Verification items for this drawing (mm, ordinates from the low corner). A direction names the side the tool comes from. Round coordinates to 2 decimals unless told otherwise and drop trailing zeros. Order: outer loops, then holes, each group sorted by start corner. A loop starts at its lowest first (then second) coordinate and runs counter-clockwise, first axis right, second up. Notation, with made-up numbers: M 17,66.25 L 42,66.25 A6 cw 42,76.25 Z; hole C -1,6 d4. An arc over 180 degrees is marked long. One line per item, written item: value. Start each with the question number.
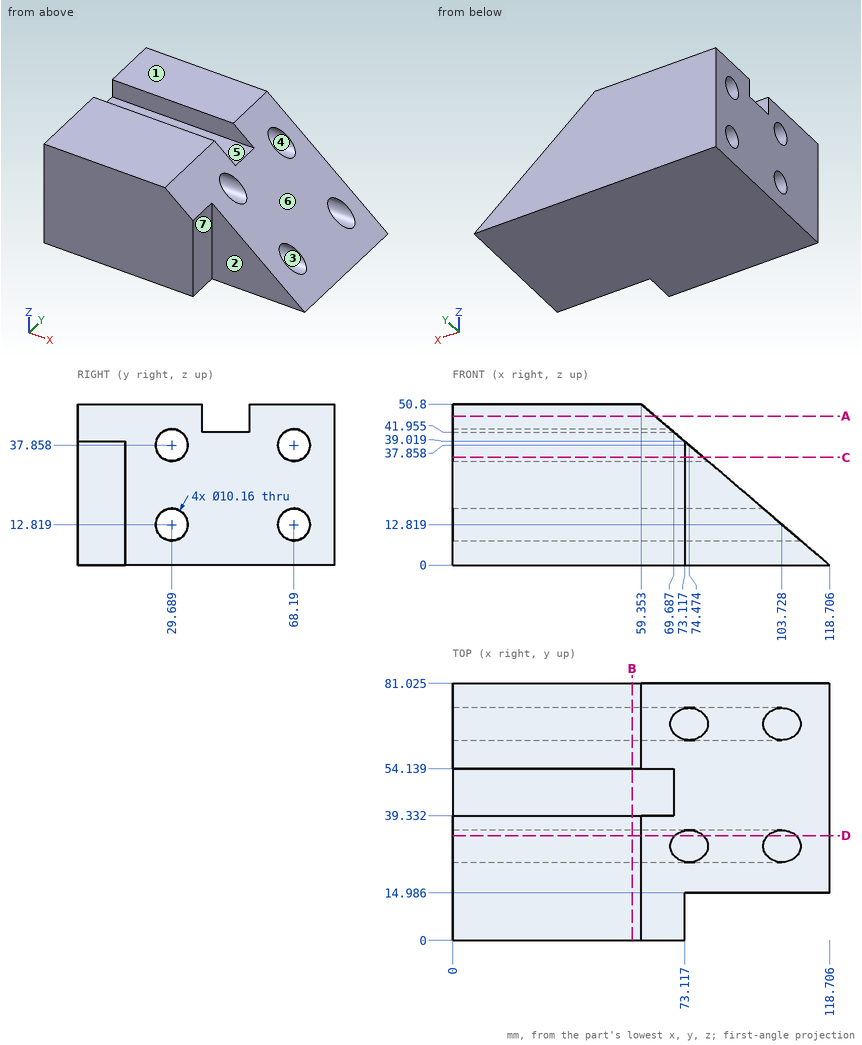
1. Section check A-A (z = 47). Record the cut outline in (x, y) (1 decimal).
2. Draft check along Z on the marked faces 1, 2, 3 and 4. Enter one of: released by +Z, released by -Z, zero draft, split by the parting line, or undercut.
3. Tool access check on the marked faces 5, 6 and 7. Record the directions out of +Z, -Z, +X, -X, +Y, -Y that give a thin tool (end or side, any length) a straight path to the whole face; none if there is none.
4. Depth check by flat-ended pin: pin 1 (19.5 mm diameter, centred on x = 90.5, z = 22.5, fed in from -Y); pin 2 (10 mm diameter, centred on x = 29, y = 29, fed in from -Z); pin 3 (2 mm diameter, centred on x = 60.5, y = 54, fed in from +Z) (1 decimal); pin 4 (1.5 mm diameter, centred on x = 84, y = 40.5, fed in from +Z) (1 decimal). Enter the tip coordinate at first touch or a pass-through.
5. Section check C-C (z = 34). Record the cut outline in (x, y) (1 decimal), and give its area (3 significant figures).
6. Scan lines: line 1 along Z through (x, y) = (37, 29) (1 decimal); line 2 along Z through (x, y) = (38.5, 70.5) (1 decimal); line 3 along X through (y, z) = (5.5, 39) (1 decimal). Record each from-to range of solid material in increasing order.
7. Section check D-D (y = 33). Record the cut outline in (x, z) (1 decimal), and give its area (3 significant figures).
8. Section check B-B (x = 56.5). Record the cut outline in (y, z) (1 decimal), and give its area (3 significant figures).
Geometry check:
1. outline: M 0,0 L 63.8,0 L 63.8,39.3 L 0,39.3 Z; M 0,54.1 L 63.8,54.1 L 63.8,81 L 0,81 Z
2. face 1: released by +Z
2. face 2: zero draft
2. face 3: undercut
2. face 4: undercut
3. face 5: +Z, +X, -X
3. face 6: +Z, +X, +Y, -Y
3. face 7: +Z, -Z, +X, -Y
4. pin 1: stops at y = 14.99
4. pin 2: stops at z = 0
4. pin 3: stops at z = 50.7
4. pin 4: stops at z = 30.3
5. outline: M 0,0 L 73.1,0 L 73.1,15 L 79,15 L 79,26.4 L 0,26.4 Z; M 0,33 L 79,33 L 79,64.9 L 0,64.9 Z; M 0,71.5 L 79,71.5 L 79,81 L 0,81 Z
5. area: 5,270 mm²
6. line 1: z = 0 to 7.8, 17.9 to 32.8, 42.9 to 50.8
6. line 2: z = 0 to 8.3, 17.3 to 33.3, 42.4 to 50.8
6. line 3: x = 0 to 73.1
7. outline: M 0,0 L 118.7,0 L 108.2,9 L 0,9 Z; M 0,16.7 L 99.2,16.7 L 79,34 L 0,34 Z; M 0,41.7 L 70,41.7 L 59.4,50.8 L 0,50.8 Z
7. area: 3,150 mm²
8. outline: M 0,0 L 81,0 L 81,50.8 L 54.1,50.8 L 54.1,42 L 39.3,42 L 39.3,50.8 L 0,50.8 Z; hole C 29.7,12.8 d10.2; hole C 29.7,37.9 d10.2; hole C 68.2,12.8 d10.2; hole C 68.2,37.9 d10.2
8. area: 3,660 mm²
